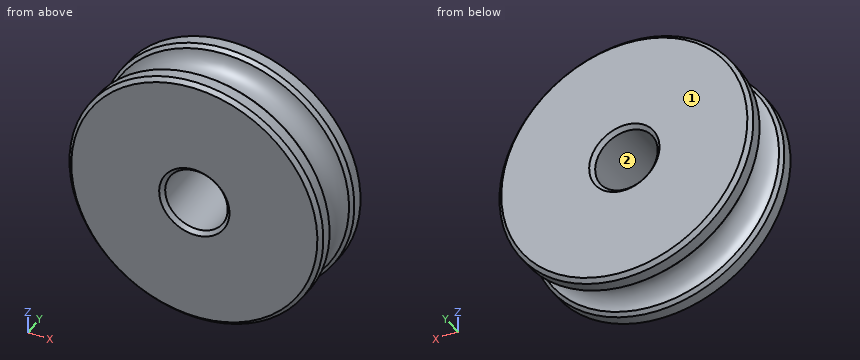
```python
from build123d import *


# Not quite as in the source:
# - a fillet or chamfer that OpenCascade refuses, or shapes differently, is made with other operations: its cross-section is extruded or revolved along the edge and cut away or added


with BuildPart() as f1:
    # F0 (on Right) → F1 (revolve)
    with BuildSketch(Plane.YZ):
        with BuildLine():
            Line((-1.975, 1.6), (0, 1.6))
            Line((0, 1.6), (1.975, 1.6))
            Line((1.975, 1.6), (1.975, 6.5))
            Line((1.975, 6.5), (1, 6.5))
            ThreePointArc((1, 6.5), (0, 5.5), (-1, 6.5))
            Line((-1, 6.5), (-1.975, 6.5))
            Line((-1.975, 6.5), (-1.975, 1.6))
        make_face()
    revolve(axis=Axis((0, 2.5333669037, 0), (0, 1, 0)))

    # F2: chamfer of 0.2 on 9 edges, made by hand

    # F2_s1 → F2_t2 (revolve, cut)
    with BuildSketch(Plane.YZ):
        Polygon((-1.775, 1.6), (-1.975, 1.8), (-1.975, 1.6), align=None)
    revolve(axis=Axis((0, -1.975, 0), (0, 1, 0)), mode=Mode.SUBTRACT)

    # F2_s3 → F2_t4 (revolve, cut)
    with BuildSketch(Plane.YZ):
        Polygon((1.775, 1.6), (1.975, 1.8), (1.975, 1.6), align=None)
    revolve(axis=Axis((0, 1.975, 0), (0, 1, 0)), mode=Mode.SUBTRACT)

    # F2_s5 → F2_t6 (revolve, cut)
    with BuildSketch(Plane.YZ):
        with BuildLine():
            Line((-0.9860132972, 6.3333333333), (-1.1832159566, 6.5))
            Line((-1.1832159566, 6.5), (-1, 6.5))
            ThreePointArc((-1, 6.5), (-0.9962551156, 6.4135376119), (-0.9860132972, 6.3333333333))
        make_face()
    revolve(axis=Axis((0, -1, 0), (0, 1, 0)), mode=Mode.SUBTRACT)

    # F2_s7 → F2_t8 (revolve, cut)
    with BuildSketch(Plane.YZ):
        Polygon((-1.775, 6.5), (-1.975, 6.3), (-1.975, 6.5), align=None)
    revolve(axis=Axis((0, -1.975, 0), (0, 1, 0)), mode=Mode.SUBTRACT)

    # F2_s9 → F2_t10 (revolve, cut)
    with BuildSketch(Plane.YZ):
        Polygon((1.975, 6.3), (1.775, 6.5), (1.975, 6.5), align=None)
    revolve(axis=Axis((0, 1.975, 0), (0, 1, 0)), mode=Mode.SUBTRACT)

    # F2_s11 → F2_t12 (revolve, cut)
    with BuildSketch(Plane.YZ):
        with BuildLine():
            Line((1.1832159566, 6.5), (0.9860132972, 6.3333333333))
            ThreePointArc((0.9860132972, 6.3333333333), (0.9962551156, 6.4135376119), (1, 6.5))
            Line((1, 6.5), (1.1832159566, 6.5))
        make_face()
    revolve(axis=Axis((0, 1, 0), (0, 1, 0)), mode=Mode.SUBTRACT)


solid = f1.part
```
Can you work these out from the model? Positions are in its coordinate system, mm. Face numbers are marked on the shaded views. Coordinates: 2 decimals unless noted, no trailing zeros. Order: outer loops, then holes, each group sorted by start corner. A loop starts at its lowest first (then second) coordinate and runs counter-clockwise, first axis right, second up.
1. If we section it at A-A (z = 0): Please give me the cut outline in (x, y) (3 decimals).
2. If we section it at B-B (x = 0): Please give me the cut outline in (y, z) (3 decimals), then the cut area to 3 significant figures.
3. If we section it at C-C (y = -1.45): Please give me the cut outline in (x, z).
4. I need wall thicknesses on line 1 (X direction, y = 0, z = -0.25); line 2 (X direction, y = 1.6, z = 0); line 3 (Y direction, x = -4, z = -4) (3 decimals). Which ranges of each line are inside material? Lowest first, please.
5. Thinking about a two-plate mould opening in Z: for the marked faces 1 and 2, which applies, +Z half, -Z half, draft (parallel to the pull), parting line (faces both ways), or undercut?
6. If we section it at D-D (y = -0.5): Please give me the cut outline in (x, z), then the cut area to 3 significant figures.
7. I'm going to push flat-ended pins straight in: pin 1 (1.5 mm diameter, centred on x = -2, y = -1, fed in from -Z); pin 2 (2.5 mm diameter, centred on x = 0, z = 0, fed in from +Y). Where does each tip first touch, or does it pass through?
Entries:
1. outline: (-6.5, -1.775) - (-6.3, -1.975) - (-1.8, -1.975) - (-1.6, -1.775) - (-1.6, 1.775) - (-1.8, 1.975) - (-6.3, 1.975) - (-6.5, 1.775) - (-6.5, 1.183) - (-6.333, 0.986) arc R1 cw to (-6.333, -0.986) - (-6.5, -1.183) - close; (1.6, -1.775) - (1.8, -1.975) - (6.3, -1.975) - (6.5, -1.775) - (6.5, -1.183) - (6.333, -0.986) arc R1 cw to (6.333, 0.986) - (6.5, 1.183) - (6.5, 1.775) - (6.3, 1.975) - (1.8, 1.975) - (1.6, 1.775) - close
2. outline: (-1.975, -6.3) - (-1.775, -6.5) - (-1.183, -6.5) - (-0.986, -6.333) arc R1 cw to (0.986, -6.333) - (1.183, -6.5) - (1.775, -6.5) - (1.975, -6.3) - (1.975, -1.8) - (1.775, -1.6) - (-1.775, -1.6) - (-1.975, -1.8) - close; (-1.975, 1.8) - (-1.775, 1.6) - (1.775, 1.6) - (1.975, 1.8) - (1.975, 6.3) - (1.775, 6.5) - (1.183, 6.5) - (0.986, 6.333) arc R1 cw to (-0.986, 6.333) - (-1.183, 6.5) - (-1.775, 6.5) - (-1.975, 6.3) - close
2. area: 35.3 mm2
3. outline: circle Ø13 at (0, 0); hole circle Ø3.2 at (0, 0)
4. line 1: x = -5.49 to -1.58, 1.58 to 5.49
4. line 2: x = -6.5 to -1.6, 1.6 to 6.5
4. line 3: y = -1.975 to -0.538, 0.538 to 1.975
5. face 1: draft
5. face 2: undercut
6. outline: circle Ø11.27 at (0, 0); hole circle Ø3.2 at (0, 0)
6. area: 91.7 mm2
7. pin 1: stops at z = -6.37
7. pin 2: passes through
